Study the drawing (mm; zero at the part's minimum x, y, z) and answer. Give positions to 0.01 mm unless a question says otherwise; leave off trailing zeros. Write each loop counter-clockwise with the first axis right and the second up, starting at its lowest first coordinate (ties: lowest second). Pieces come first, ordered by that corner, then holes. Notation, with made-up numbers: (51, 16.5) - (83, 16.5) arc R27 ccw to (83, 35.5) - close; hole circle Ø4 at (-26, -28). An arc over 180 degrees is marked (long way). Answer as CSV lines item,"result".
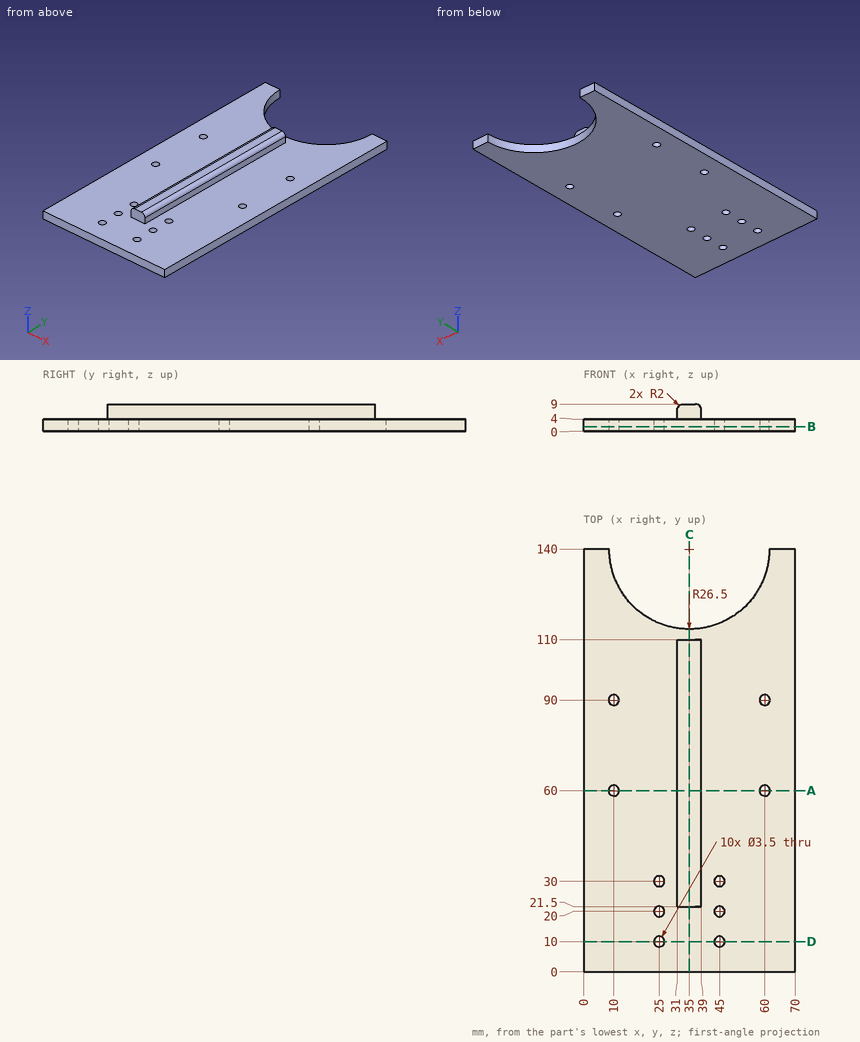
(1) A cutting plane is placed at C-C (x = 35). Write down the section's boundary in (y, z).
Worked out:
outline,"(0, 0) - (113.5, 0) - (113.5, 4) - (110, 4) - (110, 9) - (21.5, 9) - (21.5, 4) - (0, 4) - close"
(2) A cutting plane is placed at A-A (y = 60). Write down the section's boundary in (x, z), and give its area (3 significant figures).
Worked out:
outline,"(0, 0) - (8.25, 0) - (8.25, 4) - (0, 4) - close; (11.75, 0) - (58.25, 0) - (58.25, 4) - (39, 4) - (39, 7) arc R2 ccw to (37, 9) - (33, 9) arc R2 ccw to (31, 7) - (31, 4) - (11.75, 4) - close; (61.75, 0) - (70, 0) - (70, 4) - (61.75, 4) - close"
area,"290 mm^2"
(3) A cutting plane is placed at D-D (y = 10). Write down the section's boundary in (x, z).
Worked out:
outline,"(0, 0) - (23.25, 0) - (23.25, 4) - (0, 4) - close; (26.75, 0) - (43.25, 0) - (43.25, 4) - (26.75, 4) - close; (46.75, 0) - (70, 0) - (70, 4) - (46.75, 4) - close"
(4) Each of these flat-tipped pins is pushed along its axis until it touches: P1, Ø2.5, axis at y = 45, z = 6, coming from the +X side; P2, Ø5.5, axis at x = 10, y = 90, coming from the +Z side; P3, Ø2.5, axis at y = 83, z = 5.5, coming from the -X side. Where does it stop, or does it pass through?
Worked out:
P1,"stops at x = 39"
P2,"stops at z = 4"
P3,"stops at x = 31"
(5) Find the intervals of material crossed by L1, parallel to Z at x = 23.5, y = 22.5; L2, parallel to Y at x = 25, z = 2.5; L3, parallel to X at y = 66, z = 6.25, in increasing order.
Worked out:
L1,"z = 0 to 4"
L2,"y = 0 to 8.25, 11.75 to 18.25, 21.75 to 28.25, 31.75 to 115.46"
L3,"x = 31 to 39"
(6) A cutting plane is placed at B-B (z = 1.5). Count the separate pieces of the cut face and the enclosed holes in it, and give its area (3 significant figures).
Worked out:
separate pieces,"1"
enclosed holes,"10"
area,"8,600 mm^2"
